Here's how the part is built. I have some questions about the finished solid (model axes, mm). Face numbers are marked on the shaded views. A direction names the side the tool comes from. Round coordinates to 2 decimals unless told otherwise and drop trailing zeros. Order: outer loops, then holes, each group sorted by start corner. A loop starts at its lowest first (then second) coordinate and runs counter-clockwise, first axis right, second up.
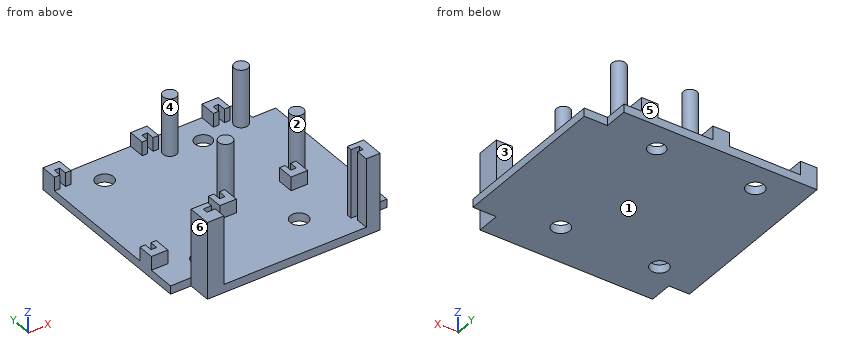
```python
from build123d import *

# Parameters (mm, degrees)
F0_R     = 3.25
F0_R_2   = 3.1
F1_DEPTH = 3
F3_DEPTH = 5
F4_DEPTH = 25
F2_R     = 2.5
F5_DEPTH = 21


with BuildPart() as f1:
    # F0 (on Top) → F1 (new body)
    with BuildSketch(Plane.XY):
        Polygon((45.104649, 50.139535), (0, 50.139535), (-25.395351, 50.139535), (-25.395351, -16.360465), (-17.895351, -16.360465), (-17.895351, -24.860465), (0, -24.860465), (45.104649, -24.860465), (45.104649, -16.360465), (53.604649, -16.360465), (53.604649, 41.639535), (45.104649, 41.639535), align=None)
        with Locations((-9.895351, -9.860465)):
            Circle(F0_R, mode=Mode.SUBTRACT)
        with Locations((26.104649, -9.860465)):
            Circle(F0_R, mode=Mode.SUBTRACT)
        with Locations((-9.895351, 40.139535)):
            Circle(F0_R, mode=Mode.SUBTRACT)
        with Locations((26.104649, 40.139535)):
            Circle(F0_R_2, mode=Mode.SUBTRACT)
    extrude(amount=F1_DEPTH)

    # F2 (on face) → F3 (join)
    with BuildSketch(Plane.XY.offset(3)):
        Polygon((-23.395351, 44.139535), (-23.395351, 47.139535), (-21.395351, 47.139535), (-21.395351, 44.139535), (-19.395351, 44.139535), (-19.395351, 50.139535), (-25.395351, 50.139535), (-25.395351, 44.139535), align=None)
        Polygon((12.604649, 50.139535), (6.604663, 50.139535), (6.604663, 44.139535), (8.604649, 44.13226), (8.604649, 47.139535), (10.604649, 47.139535), (10.604649, 44.13226), (12.604649, 44.13226), align=None)
        Polygon((8.604649, 6.639535), (8.604649, 9.639535), (6.604649, 9.639535), (6.604649, 3.639535), (12.604649, 3.639535), (12.604649, 9.639535), (10.604649, 9.639535), (10.604649, 6.639535), align=None)
        Polygon((34.604649, 6.622626), (34.604649, 9.622626), (32.604649, 9.622626), (32.604649, 3.622626), (38.604649, 3.622626), (38.604649, 9.622626), (36.604649, 9.622626), (36.604649, 6.622626), align=None)
        Polygon((-23.395351, -3.360465), (-23.395351, -0.360465), (-25.395351, -0.360465), (-25.395351, -6.360465), (-19.395351, -6.360465), (-19.395351, -0.360465), (-21.395351, -0.360465), (-21.395351, -3.360465), align=None)
        Polygon((38.604649, 50.139535), (32.604676, 50.139535), (32.604676, 44.139535), (34.604649, 44.149872), (34.604649, 47.122626), (36.604649, 47.122626), (36.604649, 44.149872), (38.604649, 44.149872), align=None)
    extrude(amount=F3_DEPTH)

    # F2 (on face) → F4 (join)
    with BuildSketch(Plane.XY.offset(3)):
        Polygon((-11.895351, -16.360465), (-17.895351, -16.360465), (-17.895351, -24.860465), (-11.895351, -24.860465), (-11.895351, -20.360465), (-14.895351, -20.360465), (-14.895351, -18.360465), (-11.895351, -18.360465), align=None)
        Polygon((40.105954, -20.360465), (40.105954, -24.860465), (45.104649, -24.860465), (45.104649, -16.360465), (39.104649, -16.360465), (39.104649, -18.360465), (42.104649, -18.360465), (42.104649, -20.360465), align=None)
    extrude(amount=F4_DEPTH)

    # F2 (on face) → F5 (join)
    with BuildSketch(Plane.XY.offset(3)):
        with Locations((14.604649, 41.139535)):
            Circle(F2_R)
        with Locations((14.604649, 12.139535)):
            Circle(F2_R)
        with Locations((40.604649, 12.139535)):
            Circle(F2_R)
        with Locations((40.604649, 41.139535)):
            Circle(F2_R)
    extrude(amount=F5_DEPTH)


solid = f1.part
```
1) I'm going to push flat-ended pins straight in: pin 1 (2.5 mm diameter, centred on x = 41, y = 41, fed in from +Z); pin 2 (12 mm diameter, centred on x = 16, z = 13.5, fed in from +Y); pin 3 (8 mm diameter, centred on x = -5, z = 18.5, fed in from +Y); pin 4 (1.5 mm diameter, centred on x = -14, z = 10, fed in from +Y). Where does each tip first touch, or does it pass through?
2) If we section it at B-B (x = 30.5): Write out the boundary of the cut face in (y, z), plus the area to 3 significant figures.
3) If we section it at C-C (y = 18): Write out the boundary of the cut face in (x, z).
4) If we section it at A-A (z = 11): Write out the boundary of the cut face in (x, y), plus the area to 3 significant figures.
5) For the marked faces 1, 2 and 3, which set-ups out of +Z, -Z, +X, -X, +Y, -Y let a thin tool reach every point of the face, with its end or its side?
6) We'd pull the mould along Y, two halves only. Please class the marked faces 4, 5 and 6: +Y half, -Y half, draft (parallel to the pull), parting line (faces both ways), or undercut.
7) I need wall thicknesses on line 1 (Y direction, x = 40.5, z = 12.5); line 2 (Y direction, x = 11.5, z = 7); line 3 (Y direction, x = 42, z = 15.25). Which ranges of each line are inside material? Lowest first, please.
Solutions:
1. pin 1: stops at z = 24
1. pin 2: stops at y = 43.64
1. pin 3: passes through
1. pin 4: stops at y = -16.36
2. outline: (-24.86, 0) - (50.14, 0) - (50.14, 3) - (-24.86, 3) - close
2. area: 225 mm2
3. outline: (-25.4, 0) - (53.6, 0) - (53.6, 3) - (-25.4, 3) - close
4. outline: (-17.9, -24.86) - (-11.9, -24.86) - (-11.9, -20.36) - (-14.9, -20.36) - (-14.9, -18.36) - (-11.9, -18.36) - (-11.9, -16.36) - (-17.9, -16.36) - close; circle Ø5 at (14.6, 12.14); circle Ø5 at (14.6, 41.14); circle Ø5 at (40.6, 12.14); circle Ø5 at (40.6, 41.14); (39.1, -18.36) - (42.1, -18.36) - (42.1, -20.36) - (40.11, -20.36) - (40.11, -24.86) - (45.1, -24.86) - (45.1, -16.36) - (39.1, -16.36) - close
4. area: 164 mm2
5. face 1: -Z, +X, -X, +Y, -Y
5. face 2: +Z
5. face 3: +Z, +X, -X
6. face 4: undercut
6. face 5: +Y half
6. face 6: draft
7. line 1: y = -24.86 to -20.36, -18.36 to -16.36, 9.64 to 14.64, 38.64 to 43.64
7. line 2: y = 3.64 to 9.64, 44.13 to 50.14
7. line 3: y = -24.86 to -20.36, -18.36 to -16.36, 10.07 to 14.21, 39.07 to 43.21
